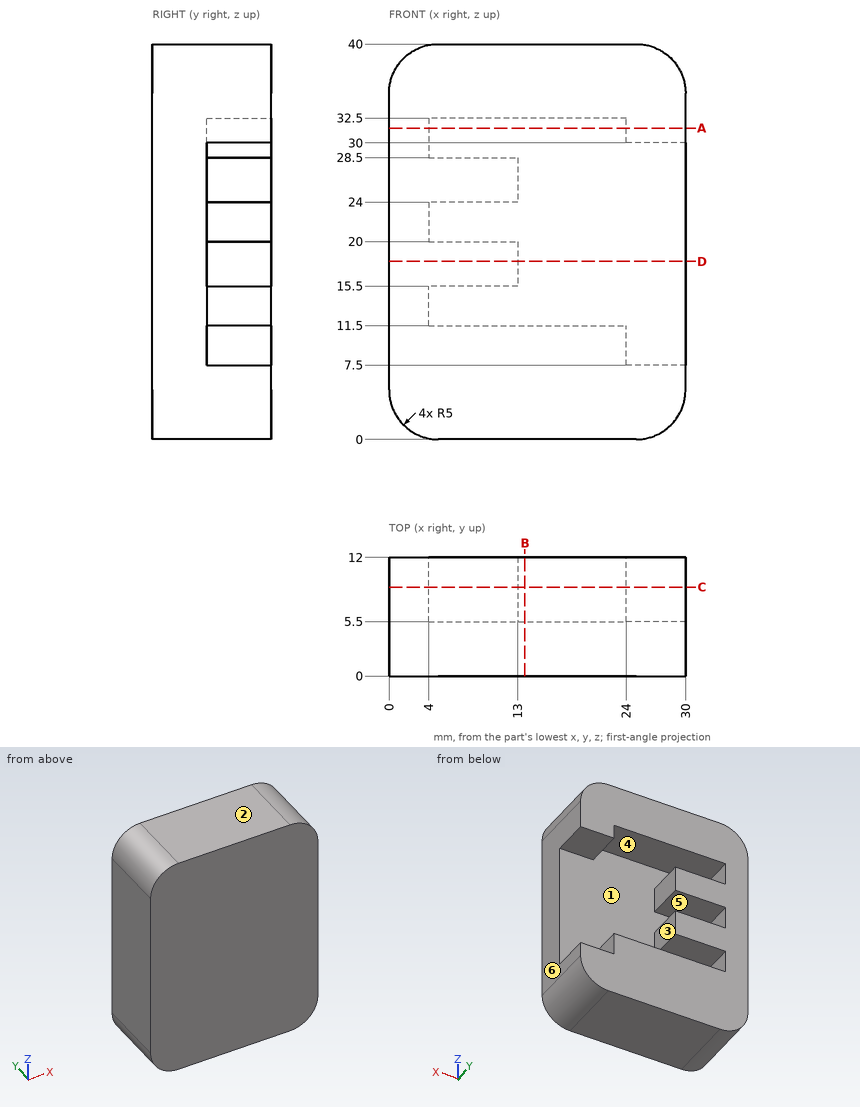
Design review of the part shown in the three views and the two pictorial views. Dimensions are in mm from the part's minimum x, y and z. A direction names the side the tool comes from. Round coordinates to 2 decimals unless told otherwise and drop trailing zeros. Order: outer loops, then holes, each group sorted by start corner. A loop starts at its lowest first (then second) coordinate and runs counter-clockwise, first axis right, second up.
Q1. Insertion check: P1, Ø5, axis at y = 9.5, z = 17.5, coming from the +X side; P2, Ø1.8, axis at x = 26.5, y = 8.5, coming from the -Z side; P3, Ø4, axis at y = 8.5, z = 12, coming from the +X side. Each pin has a flat end and moves straight along its axis. Give the tip position at first contact, or say it passes through.
Findings below:
P1: stops at x = 13
P2: stops at z = 0.04
P3: stops at x = 24
Q2. Wall thickness on line 1 (Z direction, x = 8.25, y = 9.75); line 2 (Z direction, x = 23.5, y = 6.5); line 3 (Y direction, x = 7.25, z = 22.5): over which ranges is each line inside the solid? List them lowest first.
Findings below:
line 1: z = 0 to 11.5, 15.5 to 20, 24 to 28.5, 32.5 to 40
line 2: z = 0 to 11.5, 32.5 to 40
line 3: y = 0 to 5.5
Q3. Machinability: for the marked faces 5 and 6, which of the approach directions +Z, -Z, +X, -X, +Y, -Y give a long, thin tool a straight path to every point of the face, cutting with its end or side? Answer none if there is none.
Findings below:
face 5: +X, +Y
face 6: +Z, -Z, +X, +Y, -Y
Q4. We need section B-B, the plane x = 13.75. Give the boundary of the cut face in (y, z), plus the area to 4 significant figures.
Findings below:
outline: (0, 0) - (12, 0) - (12, 11.5) - (5.5, 11.5) - (5.5, 32.5) - (12, 32.5) - (12, 40) - (0, 40) - close
area: 343.5 mm2
Q5. We need section D-D, the plane z = 18. Give the boundary of the cut face in (x, y), plus the area to 4 significant figures.
Findings below:
outline: (0, 0) - (30, 0) - (30, 5.5) - (13, 5.5) - (13, 12) - (0, 12) - close
area: 249.5 mm2
Q6. Mouldability with a two-part tool opening along X and no side actions: class the marked faces 1, 2, 3 and 4 as pulls with the +X half, pulls with the -X half, needs draft (parallel to the pull), parting line crosses it, or undercut.
Findings below:
face 1: undercut
face 2: needs draft
face 3: pulls with the +X half
face 4: undercut
Q7. We need section A-A, the plane z = 31.5. Give the boundary of the cut face in (x, y).
Findings below:
outline: (0, 0) - (30, 0) - (30, 12) - (24, 12) - (24, 5.5) - (4, 5.5) - (4, 12) - (0, 12) - close
Q8. We need section C-C, the plane y = 9. Give the boundary of the cut face in (x, z).
Findings below:
outline: (0, 5) arc R5 ccw to (5, 0) - (25, 0) arc R5 ccw to (30, 5) - (30, 7.5) - (24, 7.5) - (24, 11.5) - (4, 11.5) - (4, 15.5) - (13, 15.5) - (13, 20) - (4, 20) - (4, 24) - (13, 24) - (13, 28.5) - (4, 28.5) - (4, 32.5) - (24, 32.5) - (24, 30) - (30, 30) - (30, 35) arc R5 ccw to (25, 40) - (5, 40) arc R5 ccw to (0, 35) - close
